The listing builds one solid part. Answer for the finished solid, in the listing's coordinates (mm). Face numbers are marked on the shaded views. A direction names the side the tool comes from. Round coordinates to 2 decimals unless told otherwise and drop trailing zeros. Order: outer loops, then holes, each group sorted by start corner. A loop starts at its lowest first (then second) coordinate and runs counter-clockwise, first axis right, second up. Notation, with made-up numbers: (-36, 34) -> (18, 34) arc R21 cw to (18, 50) -> close; hole circle Ø5 at (18, 78). An arc over 180 degrees is marked (long way). Answer in a Markdown table with one row per item. Add a question column.
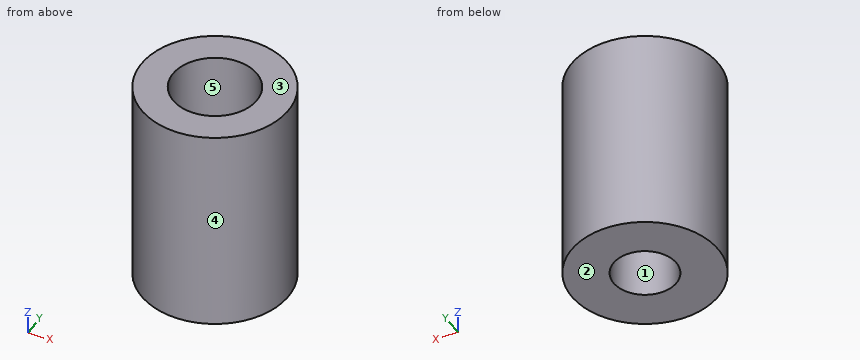
```python
from build123d import *

# Parameters (mm, degrees)
SKETCH_1_R          = 7
SKETCH_1_R_2        = 3
EXTRUDE_1_DEPTH     = 10
SKETCH_2_R          = 7
EXTRUDE_2_DEPTH     = 10
SKETCH_3_R          = 4
CUT_EXTRUDE_1_DEPTH = 8


with BuildPart() as part:
    # 草图1 → 凸台-拉伸1 (new body)
    with BuildSketch(Plane.XY):
        Circle(SKETCH_1_R)
        Circle(SKETCH_1_R_2, mode=Mode.SUBTRACT)
    extrude(amount=EXTRUDE_1_DEPTH)

    # 草图2 → 凸台-拉伸2 (add)
    with BuildSketch(Plane.XY.offset(10)):
        Circle(SKETCH_2_R)
    extrude(amount=EXTRUDE_2_DEPTH)

    # 草图3 → 切除-拉伸1 (cut)
    with BuildSketch(Plane.XY.offset(20)):
        Circle(SKETCH_3_R)
    extrude(amount=-CUT_EXTRUDE_1_DEPTH, mode=Mode.SUBTRACT)


solid = part.part
```
Item 1: The part is cut by section C-C, the plane y = -1.25. Give the vertices of the cut face in (x, z).
Item 2: For a pull along Y with two mould halves and no side action, classify the marked faces 3, 4 and 5 as released by +Y, released by -Y, zero draft, split by the parting line, or undercut.
Item 3: The part is cut by section B-B, the plane x = 2.25. Give the vertices of the cut face in (y, z).
Item 4: A tool of negligible diameter and unlimited length cuts with its end or side. For the marked faces 1 and 2, from which of +Z, -Z, +X, -X, +Y, -Y can it reach the whole face along a straight path? Write none if from no direction.
Item 5: A flat-ended cylindrical pin translates along its axis: P1, Ø1, axis at y = 2, z = 13, coming from the +X side. Find the tip coordinate at first contact, or state that the pin passes through.
Item 6: The part is cut by section A-A, the plane z = 17.25. Give the vertices of the cut face in (x, y), and give its area (3 significant figures).
Item 7: Find the intervals of material crossed by probe 1 along Y at (x, z) = (0, 16.5); probe 2 along Y at (x, z) = (0, 2.75); probe 3 along X at (y, z) = (2.25, 2), in increasing order. Write a range as [from, to].
Item 8: The part is cut by section D-D, the plane z = 3. Give the vertices of the cut face in (x, y), and give its area (3 significant figures).
Resolved:
| question | item | result |
|---|---|---|
| 1 | outline | (-6.89, 0) -> (-2.73, 0) -> (-2.73, 10) -> (2.73, 10) -> (2.73, 0) -> (6.89, 0) -> (6.89, 20) -> (3.8, 20) -> (3.8, 12) -> (-3.8, 12) -> (-3.8, 20) -> (-6.89, 20) -> close |
| 2 | face 3 | zero draft |
| 2 | face 4 | split by the parting line |
| 2 | face 5 | undercut |
| 3 | outline | (-6.63, 0) -> (-1.98, 0) -> (-1.98, 10) -> (1.98, 10) -> (1.98, 0) -> (6.63, 0) -> (6.63, 20) -> (3.31, 20) -> (3.31, 12) -> (-3.31, 12) -> (-3.31, 20) -> (-6.63, 20) -> close |
| 4 | face 1 | -Z |
| 4 | face 2 | -Z, +X, -X, +Y, -Y |
| 5 | P1 | x = 6.84 |
| 6 | outline | circle Ø14 at (0, 0); hole circle Ø8 at (0, 0) |
| 6 | area | 104 mm2 |
| 7 | probe 1 | [-7, -4], [4, 7] |
| 7 | probe 2 | [-7, -3], [3, 7] |
| 7 | probe 3 | [-6.63, -1.98], [1.98, 6.63] |
| 8 | outline | circle Ø14 at (0, 0); hole circle Ø6 at (0, 0) |
| 8 | area | 126 mm2 |
